```python
from build123d import *

# Parameters (mm, degrees)
ESTRUSIONE_ESTRUSIONE1_DEPTH         = 71
ESTRUSIONE_ESTRUSIONE5_START         = -131.7
SCHIZZO8_R                           = 46.5
ESTRUSIONE_ESTRUSIONE5_DEPTH         = 131.7
TAGLIO_ESTRUSIONE1_REACH             = 183.054
TAGLIO_ESTRUSIONE1_DIRECTION_2_REACH = 183.054
RACCORDO1_R                          = 20
TAGLIO_ESTRUSIONE2_REACH             = 188.942
SVUOTA1_START                        = -8.5
SVUOTA1_DEPTH                        = 123.2
SVUOTA1_START_2                      = 114.7
SVUOTA1_2_DEPTH                      = 5.5
ESTRUSIONE_ESTRUSIONE7_START         = 1.5
ESTRUSIONE_ESTRUSIONE7_DEPTH         = 68
ESTRUSIONE_ESTRUSIONE7_2_DEPTH       = 3
ESTRUSIONE_ESTRUSIONE7_START_2       = 66.5
ESTRUSIONE_ESTRUSIONE7_3_DEPTH       = 3
SCHIZZO15_R                          = 46.5
SCHIZZO15_R_2                        = 36.5
ESTRUSIONE_ESTRUSIONE8_DEPTH         = 20.79
ESTRUSIONE_ESTRUSIONE9_REACH         = 196.557
SCHIZZO16_R                          = 7.1


# Read off the part's stored shape, not the designer's step: Svuota1, Estrusione-Estrusione7
with BuildPart() as part:
    # Schizzo1 → Estrusione-Estrusione1 (new body)
    with BuildSketch(Plane.XY):
        with BuildLine():
            Line((11.3, 123.2), (104.3, 123.2))
            Line((104.3, 123.2), (104.3, 113.85))
            Line((104.3, 113.85), (24.875337306, -8.5))
            Line((24.875337306, -8.5), (-11.01, -8.5))
            ThreePointArc((-11.01, -8.5), (-12.511694022, -8.09709743), (-13.610030458, -6.996610042))
            Line((-13.610030458, -6.996610042), (-21.501342136, 0.894701636))
            ThreePointArc((-21.501342136, 0.894701636), (-21.856035983, 1.872259448), (-21.855688892, 2.912176215))
            Line((-21.855688892, 2.912176215), (-6.2, 91.7))
            Line((-6.2, 91.7), (-6.2, 117.7))
            Line((-6.2, 117.7), (11.3, 117.7))
            Line((11.3, 117.7), (11.3, 123.2))
        make_face()
    extrude(amount=ESTRUSIONE_ESTRUSIONE1_DEPTH)

    # Schizzo8 → Estrusione-Estrusione5 (add)
    with BuildSketch(Plane(origin=(0, 123.2, 0), x_dir=(1, 0, 0), z_dir=(0, 1, 0)).offset(ESTRUSIONE_ESTRUSIONE5_START)):
        with Locations((57.8, -35.5)):
            Circle(SCHIZZO8_R)
    extrude(amount=ESTRUSIONE_ESTRUSIONE5_DEPTH)

    # Schizzo9 → Taglio-Estrusione1 (cut, up to next)
    with BuildSketch(Plane.XY, mode=Mode.PRIVATE) as taglio_estrusione1_sk1:
        with BuildLine():
            Line((27.766685165, 6.220424861), (92.30584512, 105.64))
            add(Edge.make_bspline(
                [(92.30584512, 105.64), (97.635444472, 113.85), (104.3, 113.85)],
                knots=[0, 0, 0, 1, 1, 1], degree=2, weights=[1, 0.701406821, 1]))
            Line((104.3, 113.85), (104.3, -8.5))
            Line((104.3, -8.5), (27.766685165, -8.5))
            Line((27.766685165, -8.5), (27.766685165, 6.220424861))
        make_face()
    taglio_estrusione1_tool1 = extrude(taglio_estrusione1_sk1.sketch, amount=TAGLIO_ESTRUSIONE1_REACH, mode=Mode.PRIVATE) & part.part
    add(taglio_estrusione1_tool1.solids().sort_by_distance((76.036213, 35.53967, 0))[0], mode=Mode.SUBTRACT)

    # Schizzo9 → Taglio-Estrusione1 direction 2 (cut, up to next)
    with BuildSketch(Plane.XY, mode=Mode.PRIVATE) as taglio_estrusione1_direction_2_sk1:
        with BuildLine():
            Line((27.766685165, 6.220424861), (92.30584512, 105.64))
            add(Edge.make_bspline(
                [(92.30584512, 105.64), (97.635444472, 113.85), (104.3, 113.85)],
                knots=[0, 0, 0, 1, 1, 1], degree=2, weights=[1, 0.701406821, 1]))
            Line((104.3, 113.85), (104.3, -8.5))
            Line((104.3, -8.5), (27.766685165, -8.5))
            Line((27.766685165, -8.5), (27.766685165, 6.220424861))
        make_face()
    taglio_estrusione1_direction_2_tool1 = extrude(taglio_estrusione1_direction_2_sk1.sketch, amount=-TAGLIO_ESTRUSIONE1_DIRECTION_2_REACH, mode=Mode.PRIVATE) & part.part
    add(taglio_estrusione1_direction_2_tool1.solids().sort_by_distance((76.036213, 35.53967, 0))[0], mode=Mode.SUBTRACT)

    # Raccordo1
    # the kernel refuses this fillet: 20 mm, written as the material it takes off along each edge
    with BuildSketch(Plane(origin=(27.766685165, -8.5, -48.226424704), x_dir=(-1, 0, 0), z_dir=(0, 0, 1))) as raccordo1_piece_1:
        with BuildLine():
            CenterArc((19.290569882, -20), RACCORDO1_R, 90, 74.693720794)
            Line((0, -14.720424861), (-0.385811398, -14.614833358))
            ThreePointArc((-0.385811398, -14.614833358), (-0.4, -7.360212431), (-0.4, 0))
            Line((-0.4, 0), (0, 0.4))
            Line((0, 0.4), (19.290569882, 0.4))
            Line((19.290569882, 0.4), (19.290569882, 0))
        make_face()
    extrude(amount=167.452849408, mode=Mode.SUBTRACT)

    # Schizzo10 → Taglio-Estrusione2 (cut, up to next)
    with BuildSketch(Plane(origin=(0, 123.2, 0), x_dir=(1, 0, 0), z_dir=(0, 1, 0)), mode=Mode.PRIVATE) as taglio_estrusione2_sk1:
        with BuildLine():
            Line((104.3, 0), (87.833314835, 0))
            ThreePointArc((87.833314835, 0), (99.982929872, -15.933435984), (104.3, -35.500000151))
            Line((104.3, -35.500000151), (104.3, 0))
        make_face()
    taglio_estrusione2_tool1 = extrude(taglio_estrusione2_sk1.sketch, amount=-TAGLIO_ESTRUSIONE2_REACH, mode=Mode.PRIVATE) & part.part
    # Schizzo10 → Taglio-Estrusione2 (cut, up to next)
    with BuildSketch(Plane(origin=(0, 123.2, 0), x_dir=(1, 0, 0), z_dir=(0, 1, 0)), mode=Mode.PRIVATE) as taglio_estrusione2_sk2:
        with BuildLine():
            Line((104.3, -71), (104.3, -35.500000151))
            ThreePointArc((104.3, -35.500000151), (99.982929809, -55.066564153), (87.833314835, -71))
            Line((87.833314835, -71), (104.3, -71))
        make_face()
    taglio_estrusione2_tool2 = extrude(taglio_estrusione2_sk2.sketch, amount=-TAGLIO_ESTRUSIONE2_REACH, mode=Mode.PRIVATE) & part.part
    add(taglio_estrusione2_tool1.solids().sort_by_distance((99.557164, 123.2, 8.530088))[0], mode=Mode.SUBTRACT)
    add(taglio_estrusione2_tool2.solids().sort_by_distance((99.557164, 123.2, 62.469912))[0], mode=Mode.SUBTRACT)

    # Svuota1 outline → Svuota1 (cut)
    with BuildSketch(Plane(origin=(0, 0, 0), x_dir=(1, 0, 0), z_dir=(0, 1, 0)).offset(SVUOTA1_START)):
        with BuildLine():
            ThreePointArc((28.88633541, -68), (101.3, -35.5), (28.88633541, -3))
            Line((28.88633541, -3), (-23, -3))
            Line((-23, -3), (-23, -68))
            Line((-23, -68), (28.88633541, -68))
        make_face()
    extrude(amount=SVUOTA1_DEPTH, mode=Mode.SUBTRACT)

    # Svuota1 2 outline → Svuota1 2 (cut)
    with BuildSketch(Plane(origin=(0, 0, 0), x_dir=(1, 0, 0), z_dir=(0, 1, 0)).offset(SVUOTA1_START_2)):
        with BuildLine():
            Line((14.3, -3), (14.3, -68))
            Line((14.3, -68), (28.88633541, -68))
            ThreePointArc((28.88633541, -68), (101.3, -35.5), (28.88633541, -3))
            Line((28.88633541, -3), (14.3, -3))
        make_face()
    extrude(amount=SVUOTA1_2_DEPTH, mode=Mode.SUBTRACT)

    # Estrusione-Estrusione7 outline → Estrusione-Estrusione7 (add)
    with BuildSketch(Plane.XY.offset(ESTRUSIONE_ESTRUSIONE7_START)):
        Polygon((-6.2, 114.7), (-6.2, 116.2), (-79.280324347, 111.089725903), (-79.280324347, 108.089725903), (3.775640503, 113.897564737), (3.775640503, 114.7), align=None)
    extrude(amount=ESTRUSIONE_ESTRUSIONE7_DEPTH)

    # Estrusione-Estrusione7 2 outline → Estrusione-Estrusione7 2 (add)
    with BuildSketch(Plane.XY.offset(ESTRUSIONE_ESTRUSIONE7_START)):
        Polygon((-79.280324347, 108.089725903), (-79.280324347, 86.589725903), (3.775640503, 92.397564737), (3.775640503, 113.897564737), align=None)
    extrude(amount=ESTRUSIONE_ESTRUSIONE7_2_DEPTH)

    # Estrusione-Estrusione7 3 outline → Estrusione-Estrusione7 3 (add)
    with BuildSketch(Plane.XY.offset(ESTRUSIONE_ESTRUSIONE7_START_2)):
        Polygon((-79.280324347, 108.089725903), (-79.280324347, 86.589725903), (3.775640503, 92.397564737), (3.775640503, 113.897564737), align=None)
    extrude(amount=ESTRUSIONE_ESTRUSIONE7_3_DEPTH)

    # Schizzo15 → Estrusione-Estrusione8 (add)
    with BuildSketch(Plane(origin=(0, 123.2, 0), x_dir=(1, 0, 0), z_dir=(0, 1, 0))):
        with Locations(Location((57.8, -35.5, 0), (0, 0, 180))):
            Circle(SCHIZZO15_R)
        with Locations(Location((57.8, -35.5, 0), (0, 0, 180))):
            Circle(SCHIZZO15_R_2, mode=Mode.SUBTRACT)
    extrude(amount=ESTRUSIONE_ESTRUSIONE8_DEPTH)

    # Schizzo16 → Estrusione-Estrusione9 (add, up to next)
    with BuildSketch(Plane.XY.offset(3), mode=Mode.PRIVATE) as estrusione_estrusione9_sk1:
        Circle(SCHIZZO16_R)
    estrusione_estrusione9_tool1 = extrude(estrusione_estrusione9_sk1.sketch, amount=ESTRUSIONE_ESTRUSIONE9_REACH, mode=Mode.PRIVATE) - part.part
    add(estrusione_estrusione9_tool1.solids().sort_by_distance((0, 0, 3))[0])


solid = part.part
```
Read the model definition and answer for the solid it produces. Units are mm, in the model's axes. A direction names the side the tool comes from. Give positions to 0.01 mm unless a question says otherwise; leave off trailing zeros. Loops run counter-clockwise (first coordinate to the right, second up) from the corner with the lowest first, then second, coordinate; pieces in that order, holes last.
Item 1: Find the intervals of material crossed by line 1 along Z through (x, y) = (57.8, 129.5); line 2 along Z through (x, y) = (57.8, 89.5); line 3 along X through (y, z) = (137, 34), in increasing order.
Item 2: The part is cut by section C-C (x = 0). Write down the section's boundary in (y, z), and give its area (3 significant figures).
Item 3: The part is cut by section D-D (x = 52). Write down the section's boundary in (y, z).
Item 4: The mould has two halves that part along Y. Classify faces 4 (the flat face through (9, 114.7, 35)), 5 (the flat face through (-17.5, -3.106, 69.479)), 6 (the flat face through (16, 123.2, 61)): released by +Y, released by -Y, zero draft, split by the parting line, or undercut.
Item 5: The part is cut by section B-B (z = -5). Write down the section's boundary in (x, y).
Item 6: Each of these flat-tipped pins is pushed along its axis until it touches: pin 1 Ø8 at (x, z) = (56, 37.5) entering from -Y; pin 2 Ø8 at (x, y) = (-50, 103.5) entering from -Z; pin 3 Ø2 at (x, y) = (30.5, 115) entering from +Z. Where does it stop, or does it pass through?
Item 7: For faces 1 (the flat face through (57, 123.2, 35)), 2 (the cylindrical face through (-0.92, 7.04, 35.04)), 3 (the flat face through (-43, 102, 1.5)), determine the directions among +Z, -Z, +X, -X, +Y, -Y from which every point of the face is accessible in a straight line to the end or side of a thin tool.
Item 8: The part is cut by section A-A (y = 35). Write down the section's boundary in (x, z), and give its area (3 significant figures).
Taken from the geometry:
1. line 1: z = -11 to -1, 72 to 82
1. line 2: z = -11 to -8, 79 to 82
1. line 3: x = 11.32 to 21.33, 94.27 to 104.28
2. outline: (-8.5, 0) - (117.7, 0) - (117.7, 71) - (-8.5, 71) - (-8.5, 68) - (-7.1, 68) - (-7.1, 3) - (-8.5, 3) - close; hole (7.1, 3) - (92.13, 3) - (92.13, 4.5) - (113.63, 4.5) - (113.63, 66.5) - (92.13, 66.5) - (92.13, 68) - (7.1, 68) - close
2. area: 2,010 mm2
3. outline: (43.55, -10.64) - (143.99, -10.64) - (143.99, -0.54) - (123.2, -0.54) - (123.2, 71.54) - (143.99, 71.54) - (143.99, 81.64) - (43.55, 81.64) - (43.55, 78.61) - (120.2, 78.61) - (120.2, -7.61) - (43.55, -7.61) - close
4. face 4: undercut
4. face 5: released by -Y
4. face 6: released by +Y
5. outline: (34.95, 17.29) - (41.93, 28.03) - (41.93, 120.2) - (73.67, 120.2) - (73.67, 76.94) - (80.65, 87.68) - (80.65, 143.99) - (34.95, 143.99) - close
6. pin 1: stops at y = 120.2
6. pin 2: stops at z = 1.5
6. pin 3: stops at z = 73.85
7. face 1: +Y
7. face 2: none
7. face 3: -Z, -X, +Y
8. outline: (-16.2, 0) - (27.77, 0) arc R46.5 ccw to (46.45, -9.59) - (46.45, -6.49) arc R43.5 cw to (28.89, 3) - (-16.2, 3) - close; (-16.2, 68) - (28.89, 68) arc R43.5 cw to (46.45, 77.49) - (46.45, 80.59) arc R46.5 ccw to (27.77, 71) - (-16.2, 71) - close
8. area: 391 mm2
